Read the model definition and answer for the solid it produces. Units are mm, in the model's axes. Face numbers are marked on the shaded views. A direction names the side the tool comes from. Round coordinates to 2 decimals unless told otherwise and drop trailing zeros. Write each loop counter-clockwise with the first axis right and the second up, starting at its lowest first coordinate (ties: lowest second). Pieces come first, ordered by that corner, then holes. Notation, with made-up numbers: (-18.75, -27) - (-0.75, -27) arc R22 cw to (-0.75, -13) - close; hole circle Ø4 at (-8.75, 52). An arc over 180 degrees is marked (long way). Use one line per item in the form item = value. Start each with the question number.
1) The part is cut by section C-C, the plane z = -3.5. Give the vertices of the cut face in (x, y).
2) For the marked faces 4, 5 and 6, determine the directions among +Z, -Z, +X, -X, +Y, -Y from which every point of the face is accessible in a straight line to the end or side of a thin tool.
3) The part is cut by section B-B, the plane x = -4.5. Give the vertices of the cut face in (y, z).
4) The part is cut by section D-D, the plane y = -37.5. Give the vertices of the cut face in (x, z), plus the area to 3 significant figures.
5) For a pull along Z with two mould halves and no side action, classify the marked faces 1, 2 and 3 as released by +Z, released by -Z, zero draft, split by the parting line, or undercut.
6) The part is cut by section A-A, the plane z = 4. Give the vertices of the cut face in (x, y), plus the area to 3 significant figures.
7) Each of these flat-tipped pins is pushed along its axis until it touches: pin 1 (10 mm diameter, centred on y = -32.5, z = 3, fed in from -X); pin 2 (6.5 mm diameter, centred on x = -19.87, z = -3.5, fed in from +Y); pin 3 (6.5 mm diameter, centred on x = -0.37, y = -35.28, fed in from -Z); pin 4 (10 mm diameter, centred on x = -8.5, y = -28, fed in from -Z). Where does it stop, or does it pass through?
8) Consider line 1 along Y through (x, z) = (-4, 3); line 2 along Y through (x, z) = (-7, 3); line 3 along Z through (x, y) = (-3.5, -43). Determine where each line is inside the solid, lowest interval first. Write a range as from..to.
from build123d import *

# Parameters (mm, degrees)
SKETCH_1_W          = 23
SKETCH_1_H          = 64.4
EXTRUDE_1_DEPTH     = 8
SKETCH_3_W          = 23
SKETCH_3_H          = 64.4
SKETCH_3_R          = 5.5
EXTRUDE_2_DEPTH     = 7
SKETCH_4_W          = 23
SKETCH_4_H          = 64.4
SKETCH_4_R          = 5.5
EXTRUDE_3_DEPTH     = 7
SKETCH_5_R          = 5.5
CUT_EXTRUDE_1_DEPTH = 24
SKETCH_6_W          = 22
SKETCH_6_H          = 64.4
CUT_EXTRUDE_2_DEPTH = 11
EXTRUDE_4_DEPTH     = 9.5
SKETCH_9_R          = 5.5
CUT_EXTRUDE_3_DEPTH = 2.5


with BuildPart() as part:
    # 草圖1 → 填料-伸長1 (new body)
    with BuildSketch(Plane.XY):
        with Locations((-0.36746988, -27.579314659)):
            Rectangle(SKETCH_1_W, SKETCH_1_H)
        Polygon((9.38974967, -35.279314659), (4.511139895, -26.829314659), (-5.246079654, -26.829314659), (-10.124689429, -35.279314659), (-5.246079654, -43.729314659), (4.511139895, -43.729314659), align=None, mode=Mode.SUBTRACT)
    extrude(amount=EXTRUDE_1_DEPTH)

    # 草圖3 → 填料-伸長2 (add)
    with BuildSketch(Plane.XY.offset(8)):
        with Locations((-0.36746988, -27.579314659)):
            Rectangle(SKETCH_3_W, SKETCH_3_H)
        with Locations((-0.36746988, -35.279314659)):
            Circle(SKETCH_3_R, mode=Mode.SUBTRACT)
    extrude(amount=EXTRUDE_2_DEPTH)

    # 草圖4 → 填料-伸長3 (add)
    with BuildSketch(Plane(origin=(0, 0, 0), x_dir=(-1, 0, 0), z_dir=(0, 0, -1))):
        with Locations((0.36746988, -27.579314659)):
            Rectangle(SKETCH_4_W, SKETCH_4_H)
        with Locations((0.36746988, -35.279314659)):
            Circle(SKETCH_4_R, mode=Mode.SUBTRACT)
    extrude(amount=EXTRUDE_3_DEPTH)

    # 草圖5 → 除料-伸長1 (cut, through all)
    with BuildSketch(Plane(origin=(11.13253012, 0, 0), x_dir=(0, 0, -1), z_dir=(1, 0, 0))):
        with Locations((-4, -7.779314659)):
            Circle(SKETCH_5_R)
    extrude(amount=-CUT_EXTRUDE_1_DEPTH, mode=Mode.SUBTRACT)

    # 草圖6 → 除料-伸長2 (cut)
    with BuildSketch(Plane(origin=(11.13253012, 0, 0), x_dir=(0, 0, -1), z_dir=(1, 0, 0))):
        with Locations((-4, -27.579314659)):
            Rectangle(SKETCH_6_W, SKETCH_6_H)
    extrude(amount=-CUT_EXTRUDE_2_DEPTH, mode=Mode.SUBTRACT)

    # 草圖8 → 填料-伸長4 (add)
    with BuildSketch(Plane.XZ.offset(59.779314659)):
        Polygon((0.13253012, -7), (0.13253012, -15), (-34.36746988, -15), (-34.36746988, 32.5), (0.13253012, 32.5), align=None)
    extrude(amount=-EXTRUDE_4_DEPTH)

    # 草圖9 → 除料-伸長3 (cut)
    with BuildSketch(Plane.XZ.offset(59.779314659)):
        with Locations((-19.86746988, -3.5)):
            Circle(SKETCH_9_R)
    extrude(amount=-CUT_EXTRUDE_3_DEPTH, mode=Mode.SUBTRACT)


solid = part.part
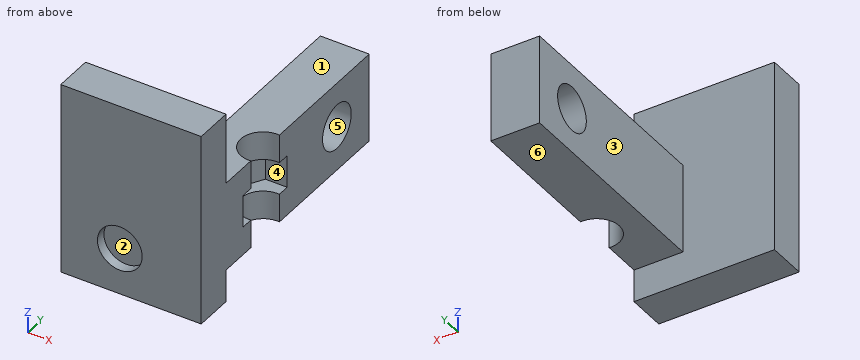
Geometry results:
q1.outline = (-34.37, -59.78) - (-25.37, -59.78) - (-25.37, -57.28) - (-14.37, -57.28) - (-14.37, -59.78) - (0.13, -59.78) - (0.13, -40.76) arc R5.5 cw (long way) to (0.13, -29.8) - (0.13, 4.62) - (-11.87, 4.62) - (-11.87, -50.28) - (-34.37, -50.28) - close
q2.face_4 = +X
q2.face_5 = +X, -X
q2.face_6 = -Z, +X, -X, +Y
q3.outline = (-59.78, -15) - (-50.28, -15) - (-50.28, -7) - (-38.91, -7) - (-38.91, 0) - (-43.73, 0) - (-43.73, 8) - (-38.91, 8) - (-38.91, 15) - (-50.28, 15) - (-50.28, 32.5) - (-59.78, 32.5) - close; (-31.65, -7) - (4.62, -7) - (4.62, 15) - (-31.65, 15) - (-31.65, 8) - (-26.83, 8) - (-26.83, 0) - (-31.65, 0) - close; hole circle Ø11 at (-7.78, 4)
q4.outline = (-11.87, -7) - (-5.4, -7) - (-5.4, 0) - (-8.84, 0) - (-8.84, 8) - (-5.4, 8) - (-5.4, 15) - (-11.87, 15) - close
q4.area = 115 mm2
q5.face_1 = released by +Z
q5.face_2 = undercut
q5.face_3 = zero draft
q6.outline = (-34.37, -59.78) - (0.13, -59.78) - (0.13, -43.73) - (-5.25, -43.73) - (-10.12, -35.28) - (-5.25, -26.83) - (0.13, -26.83) - (0.13, -13.28) - (-11.87, -13.28) - (-11.87, -50.28) - (-34.37, -50.28) - close; (-11.87, -2.28) - (0.13, -2.28) - (0.13, 4.62) - (-11.87, 4.62) - close
q6.area = 722 mm2
q7.pin_1 = -11.87
q7.pin_2 = -50.28
q7.pin_3 = through
q7.pin_4 = -7
q8.line_1 = -59.78..-43.73, -26.83..-13.19, -2.37..4.62
q8.line_2 = -59.78..-40.69, -29.87..-13.19, -2.37..4.62
q8.line_3 = -7..0, 8..15
